Build history of the part. All positions in model axes, mm. Give positions to 0.01 mm unless a question says otherwise; leave off trailing zeros. Write each loop counter-clockwise with the first axis right and the second up, starting at its lowest first coordinate (ties: lowest second). Pieces come first, ordered by that corner, then holes. Notation, with made-up numbers: M 2.25,56.5 L 55.25,56.5 A5 ccw 55.25,64.5 Z; hole C 19,14.5 d4. An arc over 180 degrees is marked long. One line per item, written item: value. Start each with the question number.
from build123d import *

# Parameters (mm, degrees)
F0_R            = 38.1
F1_DEPTH        = 7.1882
F2_R            = 11.1252
F3_DEPTH        = 7.62
F5_DEPTH        = 7.1882
F5_COPIES_COUNT = 4
F7_DEPTH        = 25.4
F9_DEPTH        = 7.1882
F10_R           = 11.90625
F11_DEPTH       = 25.4


# Not quite as in the source:
# - a pattern or mirror of a feature is missing from the dataset's text; its kind, count and spacing are read off the source's solid


with BuildPart() as f1:
    # F0 (on Front) → F1 (new body)
    with BuildSketch(Plane.XZ):
        Circle(F0_R)
    extrude(amount=F1_DEPTH)

    # F2 (on face) → F3 (cut)
    with BuildSketch(Plane.XZ.offset(7.1882)):
        Circle(F2_R)
    extrude(amount=-F3_DEPTH, mode=Mode.SUBTRACT)

    # F4 (on face) → F5 (join)
    with BuildSketch(Plane.XZ.offset(7.1882)):
        with BuildLine():
            ThreePointArc((-18.4450831863, 33.3375), (0, 19.05), (18.4450831863, 33.3375))
            ThreePointArc((18.4450831863, 33.3375), (0, 38.1), (-18.4450831863, 33.3375))
        make_face()
        with BuildLine():
            ThreePointArc((-19.05, 0), (-23.0396526434, 11.6656949), (-33.3375, 18.4450831863))
            ThreePointArc((-33.3375, 18.4450831863), (-38.1, 0), (-33.3375, -18.4450831863))
            ThreePointArc((-33.3375, -18.4450831863), (-23.0396526434, -11.6656949), (-19.05, 0))
        make_face()
        with BuildLine():
            ThreePointArc((19.05, -38.1), (18.8981657139, -35.6996182282), (18.4450831863, -33.3375))
            ThreePointArc((18.4450831863, -33.3375), (0, -38.1), (-18.4450831863, -33.3375))
            ThreePointArc((-18.4450831863, -33.3375), (-2.4003817718, -56.9981657139), (19.05, -38.1))
        make_face()
        with BuildLine():
            ThreePointArc((38.1, 0), (36.8901663726, 9.525), (33.3375, 18.4450831863))
            ThreePointArc((33.3375, 18.4450831863), (19.05, 0), (33.3375, -18.4450831863))
            ThreePointArc((33.3375, -18.4450831863), (36.8901663726, -9.525), (38.1, 0))
        make_face()
    f5 = extrude(amount=-F5_DEPTH)

    # F5_copies: F5 ×4 about axis
    f5_copies_axis = Axis((0, 0, 0), (0, 1, 0))
    for i in range(1, F5_COPIES_COUNT):
        add(f5.rotate(f5_copies_axis, i * 360 / F5_COPIES_COUNT))

    # F6 (on face) → F7 (cut)
    with BuildSketch(Plane.XZ.offset(7.1882)):
        with BuildLine():
            ThreePointArc((-33.3375, 18.4450831863), (-20.9517399354, 20.9517399354), (-18.4450831863, 33.3375))
            ThreePointArc((-18.4450831863, 33.3375), (-26.9407683632, 26.9407683632), (-33.3375, 18.4450831863))
        make_face()
        with BuildLine():
            ThreePointArc((-18.4450831863, -33.3375), (-20.9517399354, -20.9517399354), (-33.3375, -18.4450831863))
            ThreePointArc((-33.3375, -18.4450831863), (-26.9407683632, -26.9407683632), (-18.4450831863, -33.3375))
        make_face()
        with BuildLine():
            ThreePointArc((18.4450831863, -33.3375), (26.9407683632, -26.9407683632), (33.3375, -18.4450831863))
            ThreePointArc((33.3375, -18.4450831863), (20.9517399354, -20.9517399354), (18.4450831863, -33.3375))
        make_face()
        with BuildLine():
            ThreePointArc((33.3375, 18.4450831863), (26.9407683632, 26.9407683632), (18.4450831863, 33.3375))
            ThreePointArc((18.4450831863, 33.3375), (20.9517399354, 20.9517399354), (33.3375, 18.4450831863))
        make_face()
    extrude(amount=-F7_DEPTH, mode=Mode.SUBTRACT)

    # F8 (on face) → F9 (join)
    with BuildSketch(Plane.XZ.offset(7.1882)):
        with BuildLine():
            ThreePointArc((-37.1387970886, -19.0257349126), (-29.5065148582, -29.5065148582), (-19.0257349126, -37.1387970886))
            ThreePointArc((-19.0257349126, -37.1387970886), (-18.831569694, -35.2234599149), (-18.4450831863, -33.3375))
            ThreePointArc((-18.4450831863, -33.3375), (-18.0201411063, -32.0901876015), (-17.7415806811, -30.8022558951))
            ThreePointArc((-17.7415806811, -30.8022558951), (-25.1350616996, -25.1350616996), (-30.8022558951, -17.7415806811))
            ThreePointArc((-30.8022558951, -17.7415806811), (-32.0901876015, -18.0201411063), (-33.3375, -18.4450831863))
            ThreePointArc((-33.3375, -18.4450831863), (-35.2234599149, -18.831569694), (-37.1387970886, -19.0257349126))
        make_face()
        with BuildLine():
            ThreePointArc((19.0257349126, -37.1387970886), (29.5065148582, -29.5065148582), (37.1387970886, -19.0257349126))
            ThreePointArc((37.1387970886, -19.0257349126), (35.2234599149, -18.831569694), (33.3375, -18.4450831863))
            ThreePointArc((33.3375, -18.4450831863), (32.0901876015, -18.0201411063), (30.8022558951, -17.7415806811))
            ThreePointArc((30.8022558951, -17.7415806811), (25.1350616996, -25.1350616996), (17.7415806811, -30.8022558951))
            ThreePointArc((17.7415806811, -30.8022558951), (18.0201411063, -32.0901876015), (18.4450831863, -33.3375))
            ThreePointArc((18.4450831863, -33.3375), (18.831569694, -35.2234599149), (19.0257349126, -37.1387970886))
        make_face()
        with BuildLine():
            ThreePointArc((33.3375, 18.4450831863), (35.2234599149, 18.831569694), (37.1387970886, 19.0257349126))
            ThreePointArc((37.1387970886, 19.0257349126), (29.5065148582, 29.5065148582), (19.0257349126, 37.1387970886))
            ThreePointArc((19.0257349126, 37.1387970886), (18.831569694, 35.2234599149), (18.4450831863, 33.3375))
            ThreePointArc((18.4450831863, 33.3375), (18.0201411063, 32.0901876015), (17.7415806811, 30.8022558951))
            ThreePointArc((17.7415806811, 30.8022558951), (25.1350616996, 25.1350616996), (30.8022558951, 17.7415806811))
            ThreePointArc((30.8022558951, 17.7415806811), (32.0901876015, 18.0201411063), (33.3375, 18.4450831863))
        make_face()
        with BuildLine():
            ThreePointArc((-18.4450831863, 33.3375), (-18.831569694, 35.2234599149), (-19.0257349126, 37.1387970886))
            ThreePointArc((-19.0257349126, 37.1387970886), (-29.5065148582, 29.5065148582), (-37.1387970886, 19.0257349126))
            ThreePointArc((-37.1387970886, 19.0257349126), (-35.2234599149, 18.831569694), (-33.3375, 18.4450831863))
            ThreePointArc((-33.3375, 18.4450831863), (-32.0901876015, 18.0201411063), (-30.8022558951, 17.7415806811))
            ThreePointArc((-30.8022558951, 17.7415806811), (-25.1350616996, 25.1350616996), (-17.7415806811, 30.8022558951))
            ThreePointArc((-17.7415806811, 30.8022558951), (-18.0201411063, 32.0901876015), (-18.4450831863, 33.3375))
        make_face()
    extrude(amount=-F9_DEPTH)

    # F10 (on face) → F11 (cut)
    with BuildSketch(Plane.XZ.offset(7.1882)):
        with Locations((-38.1, 0)):
            Circle(F10_R)
        with Locations((0, 38.1)):
            Circle(F10_R)
        with Locations((38.1, 0)):
            Circle(F10_R)
        with Locations((0, -38.1)):
            Circle(F10_R)
    extrude(amount=-F11_DEPTH, mode=Mode.SUBTRACT)


solid = f1.part
1) Band-saw the part on B-B (x = 0). List the corners of the cut face in (y, z).
2) Band-saw the part on C-C (z = -42.5). List the corners of the cut face in (x, y), then the cut area to 3 significant figures.
3) Drop flat-ended pins along their axis: P1, Ø14.5, axis at x = 38.1, z = 0, coming from the +Y side; P2, Ø4, axis at x = 16, y = -4, coming from the -Z side; P3, Ø4, axis at x = -4.5, y = -2.5, coming from the +Z side. Give the stop position or say it passes through.
4) Band-saw the part on D-D (x = 24.5). List the corners of the cut face in (y, z), then the cut area to 3 significant figures.
5) Probe line 1 along Z through (x, y) = (0, -4.25); line 2 along Z through (x, y) = (-38, -5); line 3 along X through (y, z) = (-4.5, -28). List the from-to ranges inside material, lowest first. Write a range as from..to.
6) Band-saw the part on A-A (y = -3.5). Count the separate pieces of the cut face and the enclosed holes in it, then the cut area to 3 significant figures.
7) Mould opens along Z. For faces 1 (the face through (-25.04, -3.64, -25.23)), 2 (the face through (29.635, -3.644, 29.377)), 3 (the face through (12, -7.188, 1)) say: released by +Z, released by -Z, zero draft, split by the parting line, or undercut.
Model answer:
1. outline: M -7.19,-57.15 L 0,-57.15 L 0,-50.01 L -7.19,-50.01 Z; M -7.19,-26.19 L 0,-26.19 L 0,-11.13 L -7.19,-11.13 Z; M -7.19,11.13 L 0,11.13 L 0,26.19 L -7.19,26.19 Z; M -7.19,50.01 L 0,50.01 L 0,57.15 L -7.19,57.15 Z
2. outline: M -18.53,-7.19 L -11.06,-7.19 L -11.06,0 L -18.53,0 Z; M 11.06,-7.19 L 18.53,-7.19 L 18.53,0 L 11.06,0 Z
2. area: 107 mm²
3. P1: passes through
3. P2: stops at z = -51.02
3. P3: stops at z = 56.99
4. outline: M -7.19,-33.78 L 0,-33.78 L 0,-25.75 L -7.19,-25.75 Z; M -7.19,-18.54 L 0,-18.54 L 0,18.54 L -7.19,18.54 Z; M -7.19,25.75 L 0,25.75 L 0,33.78 L -7.19,33.78 Z
4. area: 382 mm²
5. line 1: z = -57.15..-50.01, -26.19..-11.13, 11.13..26.19, 50.01..57.15
5. line 2: z = -19.05..-11.91, 11.91..19.05
5. line 3: x = -30.94..-21.9, -17.65..-6.3, 6.3..17.65, 21.9..30.94
6. separate pieces: 1
6. enclosed holes: 9
6. area: 4,950 mm²
7. face 1: undercut
7. face 2: released by +Z
7. face 3: zero draft
